Autodesk Inventor part; units mm, degrees
ref_plane "MSC_PF1" through (0, 0, 0) normal (0, 1, 0) x (-1, 0, 0)
ref_plane "MSC_PT1" through (0, 0, 8.3331) normal (0, 0, -1) x (-1, 0, 0)
ref_plane "YZ Plane" through (0, 0, 0) normal (1, 0, 0) x (0, 1, 0)
sketch "Sketch2" plane through (0, 0, 0) normal (0, 1, 0) x (-1, 0, 0)
  line L0 (0, 8.3331) -> (0, -36.6669)
  line L1 (0, -36.6669) -> (2.5, -36.6669)
  line L2 (3, -36.1669) -> (3, -18.6669)
  line L3 (3, -18.6669) -> (2.65, -18.0607)
  line L4 (2.65, -18.0607) -> (2.65, 8.3331)
  line L5 (2.65, 8.3331) -> (0, 8.3331)
  line L6 (2.5, -36.6669) -> (3, -36.1669)
  line L7 (3, -36.6669) -> (3, -37.374)
  line L8 (0, -46.5155) -> (0, 17.4745)
  dimension "Ds" = 5.3
  dimension "NND" = 6
  dimension "b" = 18
  dimension "d3" = 30
  dimension "d5" = 45
  dimension "PTC" = 1
  dimension "NLG" = 45
revolve "Revolution1" add sketch "Sketch2" angle 360 about axis through (0, 0, 8.3331) along (0, 0, -1)
sketch "Sketch3" plane through (0, 0, 8.3331) normal (0, 0, 1) x (1, 0, 0)
  circle A0 centre (0, 0) radius 2.65
  line L0 (0, 5) -> (2.8868, 5)
  line L1 (2.8868, 5) -> (5.7735, 0)
  line L2 (5.7735, 0) -> (0, 0)
  line L3 (0, 0) -> (0, 5)
  line L4 (0, 5) -> (-2.8868, 5)
  line L5 (-2.8868, 5) -> (-5.7735, 0)
  line L6 (0, -5) -> (2.8868, -5)
  line L7 (2.8868, -5) -> (5.7735, 0)
  line L8 (-2.8868, -5) -> (-5.7735, 0)
  line L9 (0, -5) -> (-2.8868, -5)
  dimension "d9" = 60
  dimension "ParS" = 10
  dimension "msp_d11" = 10
extrude "Extrusion1" add sketch "Sketch3" along normal blind 4
sketch "Sketch4" plane through (0, 0, 0) normal (0, 1, 0) x (-1, 0, 0)
  line L0 (-5, 12.3331) -> (-5.7735, 12.3331)
  line L1 (-5.7735, 12.3331) -> (-5.7735, 11.8865)
  line L2 (-5.7735, 11.8865) -> (-5, 12.3331)
  line L3 (0, 4.4746) -> (0, 31.4838)
  line L4 (0, 27.6253) -> (0, 27.1787)
  line L5 (-5.7735, 8.3331) -> (-5.7735, 12.3331)
  line L6 (-2.8868, 12.3331) -> (-5.7735, 12.3331)
  dimension "d14" = 30
  dimension "msp_d15" = 10
revolve "Revolution2" cut sketch "Sketch4" angle 360 about axis through (0, 0, 27.6253) along (0, 0, -1)
sketch "Sketch5" plane through (0, 0, 12.3331) normal (0, 0, 1) x (1, 0, 0)
  arc A0 (4.3301, 2.5) -> (0, 5) centre (0, 0) ccw
  circle A1 centre (0, 0) radius 3.75
  dimension "d27" = 7.5
extrude "Extrusion2" cut sketch "Sketch5" against normal blind 0.8
thread "Thread1"
ref_plane "MSC_PF1" through (0, 0, 0) normal (0, 1, 0) x (-1, 0, 0)
ref_plane "MSC_PT1" through (0, 0, 8.3331) normal (0, 0, -1) x (-1, 0, 0)
fillet "Fillet1" radius 0.25 1 edges at (2.65, 0, 8.3331)
equation "\"msp_d11\" = ParS"
equation "\"msp_d15\" = ParS"
equation "\"d27\" = 0.75 * ParS"
equation "\"d28\" = 0.2 * ParK"
equation "\"d30\" = r"
equation "\"msp_d17\" = b"
equation "\"r\" = 0.25"
equation "\"THREADDIA\" = NND"
properties part number "ISO 4015 - M6 x 45" material "Stainless Steel, 440C"
For this review, take the finished solid that the model builds, in its own axes (mm). A direction names the side the tool comes from. Give positions to 0.01 mm unless a question says otherwise; leave off trailing zeros. Loops run counter-clockwise (first coordinate to the right, second up) from the corner with the lowest first, then second, coordinate; pieces in that order, holes last. Notation, with made-up numbers: M 9.5,-37.5 L 52.5,-37.5 A9 cw 52.5,-27.5 Z; hole C 42,54.5 d2. An arc over 180 degrees is marked long. Put each result on its own line as item: value. Start each with the question number.
(1) Machinability: for faces 1 (the flat face through (1, 4, 12.333)), 2 (the cylindrical face through (3, 0, -27)), which of the approach directions +Z, -Z, +X, -X, +Y, -Y give a long, thin tool a straight path to every point of the face, cutting with its end or side? Answer none if there is none.
(2) Add section A-A, the plane z = -5.5. Write out the cut boundary in (x, y), then the cut area to 3 significant figures.
(3) Wall thickness on L1, parallel to Y at x = 0, z = 11.8; L2, parallel to Z at x = -1.5, y = 1.75; L3, parallel to Z at x = 3, y = 1.25: over which ranges is each line inside the solid? List them lowest first.
(4) For pin 1 (1 mm diameter, centred on x = -1, z = -28, fed in from -Y); pin 2 (2 mm diameter, centred on x = -0.5, y = 0, fed in from +Z); pin 3 (1.5 mm diameter, centred on x = 3.5, z = -25.5, fed in from -Y), all flat-tipped, find the tip position at first contact; note any pin that passes through.
(5) The part is to be moulded in two halves that separate along X. For faces 3 (the conical face through (5.188, 0.013, 12.225)), 4 (the flat face through (0, -5, 10)), 5 (the flat face through (0, 0, 11.533)), say which applies: +X half, -X half, draft (parallel to the pull), parting line (faces both ways), or undercut.
Result:
1. face 1: +Z, +X, -X, +Y, -Y
1. face 2: -Z
2. outline: C 0,0 d5.3
2. area: 22.1 mm^2
3. L1: y = -5 to -3.75, 3.75 to 5
3. L2: z = -36.67 to 11.53
3. L3: z = 8.33 to 11.53
4. pin 1: stops at y = -2.96
4. pin 2: stops at z = 11.53
4. pin 3: stops at y = -1.2
5. face 3: +X half
5. face 4: draft
5. face 5: undercut
